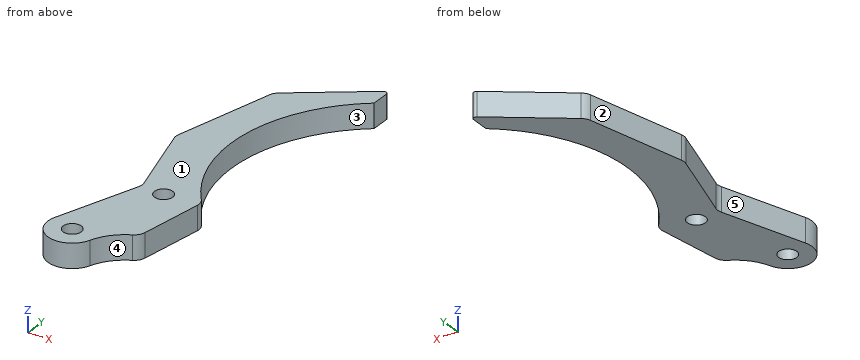
from build123d import *

# Parameters (mm, degrees)
SKETCH_1_R      = 1.5
EXTRUDE_1_DEPTH = 4


with BuildPart() as part:
    # 草图1 → 凸台-拉伸1 (new body)
    with BuildSketch(Plane.XY):
        with BuildLine():
            Line((-16.110282893, 33.654208826), (-17.814522763, 23.293438272))
            ThreePointArc((-17.814522763, 23.293438272), (-18.179793181, 22.42908037), (-18.899085656, 21.82645661))
            ThreePointArc((-18.899085656, 21.82645661), (-21.337272658, 19.958522776), (-22.891934151, 17.309568206))
            ThreePointArc((-22.891934151, 17.309568206), (-27.990948412, 14.860061819), (-30.440454799, 19.959076079))
            Line((-30.440454799, 19.959076079), (-25.681476272, 33.517536514))
            ThreePointArc((-25.681476272, 33.517536514), (-25.569637864, 34.115664062), (-25.6428361, 34.719738902))
            Line((-25.6428361, 34.719738902), (-29.24172024, 47.558366666))
            ThreePointArc((-29.24172024, 47.558366666), (-29.31581841, 48.075186607), (-29.253628902, 48.593574353))
            Line((-29.253628902, 48.593574353), (-25.108232608, 64.808221419))
            ThreePointArc((-25.108232608, 64.808221419), (-24.821945701, 65.441071196), (-24.336476636, 65.937839573))
            Line((-24.336476636, 65.937839573), (-12.719407819, 74.272976396))
            ThreePointArc((-12.719407819, 74.272976396), (-12.199607619, 74.311552327), (-11.927927269, 73.866726364))
            Line((-11.927927269, 73.866726364), (-11.927927269, 70.840856193))
            ThreePointArc((-11.927927269, 70.840856193), (-21.765630275, 54.0055336), (-16.519844581, 35.225485153))
            ThreePointArc((-16.519844581, 35.225485153), (-16.148427264, 34.483281689), (-16.110282893, 33.654208826))
        make_face()
        with Locations((-26.666194475, 18.634322143)):
            Circle(SKETCH_1_R, mode=Mode.SUBTRACT)
        with Locations((-21.666194475, 33.634322143)):
            Circle(SKETCH_1_R, mode=Mode.SUBTRACT)
    extrude(amount=EXTRUDE_1_DEPTH)


solid = part.part
Can you work these out from the model? Positions are in its coordinate system, mm. Face numbers are marked on the shaded views. A direction names the side the tool comes from. Round coordinates to 2 decimals unless told otherwise and drop trailing zeros. Write each loop counter-clockwise with the first axis right and the second up, starting at its lowest first coordinate (ties: lowest second). Pieces come first, ordered by that corner, then holes. Notation, with made-up numbers: M 10.5,69.5 L 53.5,69.5 A33 ccw 53.5,108.5 Z; hole C 70,76 d6. An arc over 180 degrees is marked long. Use a Markdown table: item, result.
Item 1: I want a section at C-C (x = -15.5). List the corners of the cut face in (y, z) for me.
Found:
| item | result |
|---|---|
| outline | M 67.59,0 L 72.28,0 L 72.28,4 L 67.59,4 Z |
Item 2: We'd pull the mould along Y, two halves only. Please class the marked faces 1, 2 and 3: released by +Y, released by -Y, zero draft, split by the parting line, or undercut.
Found:
| item | result |
|---|---|
| face 1 | zero draft |
| face 2 | released by +Y |
| face 3 | undercut |
Item 3: I want a section at A-A (z = 1.4). List the corners of the cut face in (x, y) for me.
Found:
| item | result |
|---|---|
| outline | M -30.44,19.96 A4 ccw -22.89,17.31 A8 cw -18.9,21.83 A2 ccw -17.81,23.29 L -16.11,33.65 A2 ccw -16.52,35.23 A25 cw -11.93,70.84 L -11.93,73.87 A0.5 ccw -12.72,74.27 L -24.34,65.94 A2 ccw -25.11,64.81 L -29.25,48.59 A2 ccw -29.24,47.56 L -25.64,34.72 A2 cw -25.68,33.52 Z; hole C -26.67,18.63 d3; hole C -21.67,33.63 d3 |
Item 4: For pin 1 Ø1.5 at (x, z) = (-17.5, 3) entering from -Y, with a flat end and sliding along its axis, tell me the tip position at first contact or that it passes through.
Found:
| item | result |
|---|---|
| pin 1 | stops at y = 22.34 |
Item 5: I want a section at B-B (y = 69.5). List the corners of the cut face in (x, z) for me, and give its area (3 significant figures).
Found:
| item | result |
|---|---|
| outline | M -19.37,0 L -13.57,0 L -13.57,4 L -19.37,4 Z |
| area | 23.2 mm2 |
Item 6: If I drill on line 1 along Y through (x, z) = (-18.25, 2.45); line 2 along Y through (x, z) = (-22.25, 2.95); line 3 along Y through (x, z) = (-24.25, 2.95), over which ranges is the centre line in solid material (lowest first)? Write a range as [from, to].
Found:
| item | result |
|---|---|
| line 1 | y = [22.34, 37.69], [63.93, 70.3] |
| line 2 | y = [18.7, 32.25], [35.02, 67.43] |
| line 3 | y = [15.45, 66] |
Item 7: Which directions (+Z, -Z, +X, -X, +Y, -Y) give clear straight access to the entire face, cutting with the end or side of a thin tool? Please do the marked faces 4 and 5.
Found:
| item | result |
|---|---|
| face 4 | +Z, -Z, +X, -Y |
| face 5 | +Z, -Z, -X |
